```python
from build123d import *

# Parameters (mm, degrees)
SKETCH1_R           = 6
SKETCH1_R_2         = 3.175
BOSS_EXTRUDE1_DEPTH = 16
SKETCH2_R           = 30
BOSS_EXTRUDE2_DEPTH = 5
BOSS_EXTRUDE3_DEPTH = 6


with BuildPart() as part:
    # Sketch1 → Boss-Extrude1 (new body)
    with BuildSketch(Plane(origin=(0, 0, 0), x_dir=(1, 0, 0), z_dir=(0, 1, 0))):
        with Locations(Location((0, 0, 0), (0, 0, 270))):
            Circle(SKETCH1_R)
        with Locations(Location((0, 0, 0), (0, 0, 270))):
            Circle(SKETCH1_R_2, mode=Mode.SUBTRACT)
    extrude(amount=BOSS_EXTRUDE1_DEPTH)

    # Sketch2 → Boss-Extrude2 (add)
    with BuildSketch(Plane(origin=(0, 16, 0), x_dir=(1, 0, 0), z_dir=(0, 1, 0))):
        with Locations(Location((0, 0, 0), (0, 0, 270))):
            Circle(SKETCH2_R)
    extrude(amount=BOSS_EXTRUDE2_DEPTH)

    # Sketch3 → Boss-Extrude3 (add)
    with BuildSketch(Plane(origin=(0, 21, 0), x_dir=(1, 0, 0), z_dir=(0, 1, 0))):
        with BuildLine():
            Line((17.633557569, -24.270509831), (176.335575688, -242.705098312))
            ThreePointArc((176.335575688, -242.705098312), (0, -300), (-176.335575688, -242.705098312))
            Line((-176.335575688, -242.705098312), (-17.633557569, -24.270509831))
            ThreePointArc((-17.633557569, -24.270509831), (0, 30), (17.633557569, -24.270509831))
        make_face()
    extrude(amount=BOSS_EXTRUDE3_DEPTH)


solid = part.part
```
The listing builds one solid part. Answer for the finished solid, in the listing's coordinates (mm). A direction names the side the tool comes from. Coordinates: 2 decimals unless noted, no trailing zeros. Loops run counter-clockwise (first coordinate to the right, second up) from the corner with the lowest first, then second, coordinate; pieces in that order, holes last. Notation, with made-up numbers: (0.25, 30) - (50.25, 30) arc R14 ccw to (50.25, 38) - close; hole circle Ø1 at (-19, 18). An arc over 180 degrees is marked (long way). Use a Markdown table: item, result. Add a question column.
1) The part is cut by section A-A, the plane y = 9.25. Give the vertices of the cut face in (x, z) (3 decimals).
2) The part is cut by section C-C, the plane x = 40.5. Give the vertices of the cut face in (y, z), and give its area (3 significant figures).
3) For faces 1 (the flat face through (-3, 0, 3)), 2 (the cylindrical face through (1.802, 7.888, 5.723)), determine the directions among +Z, -Z, +X, -X, +Y, -Y from which every point of the face is accessible in a straight line to the end or side of a thin tool.
4) The part is cut by section B-B, the plane z = 255. Give the vertices of the cut face in (x, y), and give its area (3 significant figures).
5) Given pin 1 (3 mm diameter, centred on x = 13, y = 19, fed in from +Z); pin 2 (3 mm diameter, centred on y = 20, z = 182.5, fed in from -X); pin 3 (10 mm diameter, centred on x = -37, y = 18.5, fed in from -Z), each flat-ended and moving along its own axis, determine where each tip first touches the part or whether it passes through.
6) Find the intervals of material crossed by line 1 (X direction, y = 9.75, z = 0) (3 decimals); line 2 (Y direction, x = 12.5, z = 206); line 3 (Y direction, x = 5, z = -4.5), in increasing order.
Here are the results:
| question | item | result |
|---|---|---|
| 1 | outline | circle Ø12 at (0, 0); hole circle Ø6.35 at (0, 0) |
| 2 | outline | (21, 55.74) - (27, 55.74) - (27, 297.25) - (21, 297.25) - close |
| 2 | area | 1,450 mm^2 |
| 3 | face 1 | +Z, -Z, +X, -X, -Y |
| 3 | face 2 | -Y |
| 4 | outline | (-158.03, 21) - (158.03, 21) - (158.03, 27) - (-158.03, 27) - close |
| 4 | area | 1,900 mm^2 |
| 5 | pin 1 | stops at z = 27.71 |
| 5 | pin 2 | stops at x = -133.41 |
| 5 | pin 3 | stops at z = 44.97 |
| 6 | line 1 | x = -6 to -3.175, 3.175 to 6 |
| 6 | line 2 | y = 21 to 27 |
| 6 | line 3 | y = 16 to 27 |
